from build123d import *

# Parameters (mm, degrees)
SKETCH1_R           = 13.97
SKETCH1_R_2         = 8.89
BOSS_EXTRUDE1_DEPTH = 4.826
SKETCH2_R           = 13.97
BOSS_EXTRUDE2_DEPTH = 5.08
SKETCH3_R           = 1.7145
BOSS_EXTRUDE3_DEPTH = 3.81


with BuildPart() as part:
    # Sketch1 → Boss-Extrude1 (new body)
    with BuildSketch(Plane(origin=(0, 0, 0), x_dir=(1, 0, 0), z_dir=(0, 1, 0))):
        with Locations(Location((0, 0, 0), (0, 0, 270))):  # turned: the seam where the file's is
            Circle(SKETCH1_R)
        with Locations(Location((0, 0, 0), (0, 0, 270))):  # turned: the seam where the file's is
            Circle(SKETCH1_R_2, mode=Mode.SUBTRACT)
    extrude(amount=BOSS_EXTRUDE1_DEPTH)

    # Sketch2 → Boss-Extrude2 (add)
    with BuildSketch(Plane(origin=(0, 4.826, 0), x_dir=(1, 0, 0), z_dir=(0, 1, 0))):
        with Locations(Location((0, 0, 0), (0, 0, 270))):  # turned: the seam where the file's is
            Circle(SKETCH2_R)
    extrude(amount=BOSS_EXTRUDE2_DEPTH)

    # Sketch3 → Boss-Extrude3 (add, symmetric)
    with BuildSketch(Plane.XY):
        with BuildLine():
            Line((-5.08, 9.906), (-5.08, 14.986))
            ThreePointArc((-5.08, 14.986), (0, 20.066), (5.08, 14.986))
            Line((5.08, 14.986), (5.08, 9.906))
            Line((5.08, 9.906), (-5.08, 9.906))
        make_face()
        with Locations((0, 14.986)):
            Circle(SKETCH3_R, mode=Mode.SUBTRACT)
    extrude(amount=BOSS_EXTRUDE3_DEPTH, both=True)


solid = part.part
The listing builds one solid part. Answer for the finished solid, in the listing's coordinates (mm). A direction names the side the tool comes from. Round coordinates to 2 decimals unless told otherwise and drop trailing zeros. Write each loop counter-clockwise with the first axis right and the second up, starting at its lowest first coordinate (ties: lowest second). Pieces come first, ordered by that corner, then holes. Notation, with made-up numbers: M 87,-8 L 128,-8 A21 cw 128,5 Z; hole C 14,-35.75 d7. An arc over 180 degrees is marked long. Write each question's results on one line, items separated by ' | '. Start each with the question number.
(1) The part is cut by section D-D, the plane y = 2.5. Write down the section's boundary in (x, z).
(2) The part is cut by section A-A, the plane x = 0. Write down the section's boundary in (y, z).
(3) Find the intervals of material crossed by line 1 (X direction, y = 2.55, z = 0); line 2 (Y direction, x = 0, z = 0.75); line 3 (X direction, y = 2.5, z = 1.25), in increasing order.
(4) Determine the mould class of faces 6 (the flat face through (0, 4.826, 0)), 7 (the flat face through (-5.08, 12, 0)), 8 (the cylindrical face through (-0.112, 20.065, 0.053)) for opening direction X: +X half, -X half, draft (parallel to the pull), parting line (faces both ways), or undercut.
(5) Each of these flat-tipped pins is pushed along its axis until it touches: P1, Ø10, axis at y = 12, z = -6.5, coming from the +X side; P2, Ø12, axis at x = -8, y = 16, coming from the +Z side; P3, Ø8, axis at x = -6.5, y = 4, coming from the -Z side. Where does it stop, or does it pass through?
(6) For faces 1 (the flat face through (0, 13, 3.81)), 2 (the flat face through (0, 13, -3.81)), 3 (the cylindrical face through (-8.68, 2.38, -1.93)), 4 (the cylindrical face through (13.85, 4.88, -1.82)), 5 (the flat face through (5.08, 12, 0)), determine the directions among +Z, -Z, +X, -X, +Y, -Y from which every point of the face is accessible in a straight line to the end or side of a thin tool.
(7) The part is cut by section C-C, the plane y = 14. Write down the section's boundary in (x, z).
(8) The part is cut by section B-B, the plane z = 0. Write down the section's boundary in (x, y), and give its area (3 significant figures).
Worked answers:
1) outline: C 0,0 d27.94; hole C 0,0 d17.78
2) outline: M 0,-13.97 L 9.91,-13.97 L 9.91,-3.81 L 13.27,-3.81 L 13.27,3.81 L 9.91,3.81 L 9.91,13.97 L 0,13.97 L 0,8.89 L 4.83,8.89 L 4.83,-8.89 L 0,-8.89 Z; M 16.7,-3.81 L 20.07,-3.81 L 20.07,3.81 L 16.7,3.81 Z
3) line 1: x = -13.97 to -8.89, 8.89 to 13.97 | line 2: y = 4.83 to 13.27, 16.7 to 20.07 | line 3: x = -13.91 to -8.8, 8.8 to 13.91
4) face 6: undercut | face 7: -X half | face 8: parting line
5) P1: stops at x = 13.83 | P2: stops at z = 3.81 | P3: stops at z = -13.74
6) face 1: +Z, +X, -X, +Y | face 2: -Z, +X, -X, +Y | face 3: -Y | face 4: +Y, -Y | face 5: +Z, -Z, +X, +Y
7) outline: M -5.08,-3.81 L -1.4,-3.81 L -1.4,3.81 L -5.08,3.81 Z; M 1.4,-3.81 L 5.08,-3.81 L 5.08,3.81 L 1.4,3.81 Z
8) outline: M -13.97,0 L -8.89,0 L -8.89,4.83 L 8.89,4.83 L 8.89,0 L 13.97,0 L 13.97,9.91 L 5.08,9.91 L 5.08,14.99 A5.08 ccw -5.08,14.99 L -5.08,9.91 L -13.97,9.91 Z; hole C 0,14.99 d3.43 | area: 274 mm²
